CAD build for the part. Positions are in the model's coordinates, mm. A direction names the side the tool comes from. Coordinates: 2 decimals unless noted, no trailing zeros. Write each loop counter-clockwise with the first axis right and the second up, starting at its lowest first coordinate (ties: lowest second). Pieces come first, ordered by that corner, then holes. Notation, with made-up numbers: (-7, -23) - (21, -23) arc R23 cw to (21, 15) - close; hole circle Ø10 at (-6.75, -33). An arc over 180 degrees is marked (long way). Answer in a Markdown table with one row per item. Add a question column.
Q1. Band-saw the part on B-B (z = 16.25). List the corners of the cut face in (x, y).
Q2. 3-axis set-ups, long thin cutter, end or side, ignore diameter. For faces 4 (the flat face through (-1.016, -4, 14)), 5 (the flat face through (0, 3.2, 25.4)): which of +Z, -Z, +X, -X, +Y, -Y reach the whole face in a straight line?
Q3. Band-saw the part on A-A (z = 21). List the corners of the cut face in (x, y).
Q4. Pin check, flat tips, straight feed: pin 1 (1.5 mm diameter, centred on y = 2, z = 22, fed in from +X); pin 2 (2 mm diameter, centred on x = -0.5, z = 18, fed in from +Y); pin 3 (2 mm diameter, centred on x = -14, y = 14, fed in from +Z); pin 4 (2 mm diameter, centred on y = 8, z = 21.5, fed in from -X). Stop position of each tip, or through.
Q5. Drill centre lines: line 1 along X through (y, z) = (-3.5, 16.75); line 2 along X through (y, z) = (0, 20.5); line 3 along Z through (x, y) = (10, 14). Where is each one in solid material? Low to high. Write a range as from..to.
Q6. Two-plate mould, pull along Y, no slides. Class faces 1 (the conical face through (-1.77, -7.98, 15.81)), 2 (the flat face through (1.016, 4, 14)), 3 (the flat face through (-7, 16, 2.032)): +Y half, -Y half, draft (parallel to the pull), parting line (faces both ways), or undercut.
```python
from build123d import *

# Parameters (mm, degrees)
F0_W     = 6.096
F0_H     = 6.35
F2_R     = 5.08
F3_DEPTH = 24.13
F4_R     = 2.54
F5_W     = 2.032
F5_H     = 2.54
F6_DEPTH = 25.4


with BuildPart() as f1:
    # F0 (on Front) → F1 (revolve)
    with BuildSketch(Plane.XZ):
        Polygon((0, 19.05), (0, 0), (19.05, 0), (19.05, 2.032), (17.018, 2.032), (6.096, 19.05), align=None)
        with Locations((3.048, 22.225)):
            Rectangle(F0_W, F0_H)
    revolve(axis=Axis((0, 0, 9.525), (0, 0, 1)))

    # F2 (on face) → F3 (cut)
    with BuildSketch(Plane.XY.offset(25.4)):
        Circle(F2_R)
    extrude(amount=-F3_DEPTH, mode=Mode.SUBTRACT)

    # F4
    f4_edges = [f1.edges().sort_by_distance(p)[0] for p in [
        (-6.096, 0, 19.05),
    ]]
    fillet(f4_edges, radius=F4_R)

    # F5 (on face) → F6 (join)
    with BuildSketch(Plane.XY.offset(25.4)):
        with Locations((0, -4.318)):
            Rectangle(F5_W, F5_H)
        with Locations((0, 4.318)):
            Rectangle(F5_W, F5_H)
    extrude(amount=-F6_DEPTH)


solid = f1.part
```
Checked values:
| question | item | result |
|---|---|---|
| 1 | outline | circle Ø15.79 at (0, 0); hole (-1.02, -4.98) - (-1.02, -3.05) - (1.02, -3.05) - (1.02, -4.98) arc R5.08 ccw to (1.02, 4.98) - (1.02, 3.05) - (-1.02, 3.05) - (-1.02, 4.98) arc R5.08 ccw to start |
| 2 | face 4 | +Z |
| 2 | face 5 | +Z, +X, -X, +Y, -Y |
| 3 | outline | circle Ø12.19 at (0, 0); hole (-1.02, -4.98) - (-1.02, -3.05) - (1.02, -3.05) - (1.02, -4.98) arc R5.08 ccw to (1.02, 4.98) - (1.02, 3.05) - (-1.02, 3.05) - (-1.02, 4.98) arc R5.08 ccw to start |
| 4 | pin 1 | stops at x = 5.97 |
| 4 | pin 2 | stops at y = 7.4 |
| 4 | pin 3 | stops at z = 2.03 |
| 4 | pin 4 | passes through |
| 5 | line 1 | x = -6.71..-3.68, -1.02..1.02, 3.68..6.71 |
| 5 | line 2 | x = -6.1..-5.08, 5.08..6.1 |
| 5 | line 3 | z = 0..2.03 |
| 6 | face 1 | parting line |
| 6 | face 2 | undercut |
| 6 | face 3 | draft |
